Work out the finished part from the listing and answer in its coordinate system (mm). Face numbers are marked on the shaded views. A direction names the side the tool comes from. Coordinates: 2 decimals unless noted, no trailing zeros. Write each loop counter-clockwise with the first axis right and the second up, starting at its lowest first coordinate (ties: lowest second). Pieces come first, ordered by that corner, then holes. Notation, with made-up numbers: M -28.75,34.5 L 20.25,34.5 A24 ccw 20.25,61.5 Z; hole C 76.5,-4.75 d1. An arc over 180 degrees is marked long. Answer as CSV lines item,"result". Start each with the question number.
(1) The mould has two halves that part along X. Classify the marked faces 5, 6, 7 and 8: released by +X, released by -X, zero draft, split by the parting line, or undercut.
(2) Find the intervals of material crossed by L1, parallel to Y at x = -472, z = 61.5; L2, parallel to X at y = 260.5, z = 361; L3, parallel to Y at x = -29.5, z = 273, in increasing order. Write a range as [from, to].
(3) Flat-ended cylindrical pins translate along their axes: P1, Ø1.5, axis at x = -123.5, y = 183.5, coming from the -Z side; P2, Ø8, axis at x = -273.5, z = 408.5, coming from the +Y side; P3, Ø12, axis at y = 246.5, z = 200, coming from the +X side. Find the tip coordinate at first contact, or state that the pin passes through.
(4) For the marked faces 1, 2, 3 and 4, determine the directions among +Z, -Z, +X, -X, +Y, -Y from which every point of the face is accessible in a straight line to the end or side of a thin tool.
(5) A cutting plane is placed at D-D on x = -546. Give the vertices of the cut face in (y, z), then the cut area to 3 significant figures.
(6) A cutting plane is placed at A-A on z = 421. Give the vertices of the cut face in (x, y).
(7) A cutting plane is placed at B-B on y = 156.5. Give the vertices of the cut face in (x, z).
(8) A cutting plane is placed at C-C on x = -83. Give the vertices of the cut face in (y, z).
from build123d import *

# Parameters (mm, degrees)
F0_W      = 762
F0_H      = 457.2
F1_DEPTH  = 25.4
F2_W      = 50.8
F2_H      = 457.2
F3_DEPTH  = 25.4
F4_W      = 762
F4_H      = 457.2
F4_W_2    = 711.2
F4_H_2    = 406.4
F5_DEPTH  = 457.2
F6_W      = 50.8
F6_H      = 482.6
F7_DEPTH  = 25.4
F8_W      = 50.8
F8_H      = 482.6
F9_DEPTH  = 25.4
F10_W     = 76.2
F10_H     = 482.6
F11_DEPTH = 25.4
F12_W     = 76.2
F12_H     = 482.6
F13_DEPTH = 25.4
F15_DEPTH = 25.4


with BuildPart() as f1:
    # F0 (on Top) → F1 (new body)
    with BuildSketch(Plane.XY):
        with Locations((-381, 228.6)):
            Rectangle(F0_W, F0_H)
    extrude(amount=F1_DEPTH)

    # F2 (on face) → F3 (join)
    with BuildSketch(Plane(origin=(0, 0, 0), x_dir=(1, 0, 0), z_dir=(0, 0, -1))):
        with Locations((-584.2, -228.6)):
            Rectangle(F2_W, F2_H)
        with Locations((-177.8, -228.6)):
            Rectangle(F2_W, F2_H)
    extrude(amount=F3_DEPTH)

    # F4 (on face) → F5 (join)
    with BuildSketch(Plane.XY.offset(25.4)):
        with Locations((-381, 228.6)):
            Rectangle(F4_W, F4_H)
        with Locations((-381, 228.6)):
            Rectangle(F4_W_2, F4_H_2, mode=Mode.SUBTRACT)
    extrude(amount=F5_DEPTH)

    # F6 (on face) → F7 (join)
    with BuildSketch(Plane(origin=(0, 457.2, 0), x_dir=(-1, 0, 0), z_dir=(0, 1, 0))):
        with Locations((25.4, 241.3)):
            Rectangle(F6_W, F6_H)
        with Locations((736.6, 241.3)):
            Rectangle(F6_W, F6_H)
    extrude(amount=F7_DEPTH)

    # F8 (on face) → F9 (join)
    with BuildSketch(Plane.XZ):
        with Locations((-736.6, 241.3)):
            Rectangle(F8_W, F8_H)
        with Locations((-25.4, 241.3)):
            Rectangle(F8_W, F8_H)
    extrude(amount=F9_DEPTH)

    # F10 (on face) → F11 (join)
    with BuildSketch(Plane.YZ):
        with Locations((12.7, 241.3)):
            Rectangle(F10_W, F10_H)
        with Locations((444.5, 241.3)):
            Rectangle(F10_W, F10_H)
    extrude(amount=F11_DEPTH)

    # F12 (on face) → F13 (join)
    with BuildSketch(Plane(origin=(-762, 0, 0), x_dir=(0, -1, 0), z_dir=(-1, 0, 0))):
        with Locations((-444.5, 241.3)):
            Rectangle(F12_W, F12_H)
        with Locations((-12.7, 241.3)):
            Rectangle(F12_W, F12_H)
    extrude(amount=F13_DEPTH)

    # F14 (on face) → F15 (cut)
    with BuildSketch(Plane.XZ):
        with BuildLine():
            Line((-635, 482.6), (-635, 463.55))
            ThreePointArc((-635, 463.55), (-629.420384, 450.079616), (-615.95, 444.5))
            Line((-615.95, 444.5), (-146.05, 444.5))
            ThreePointArc((-146.05, 444.5), (-132.579616, 450.079616), (-127, 463.55))
            Line((-127, 463.55), (-127, 482.6))
            Line((-127, 482.6), (-635, 482.6))
        make_face()
    extrude(amount=-F15_DEPTH, mode=Mode.SUBTRACT)


solid = f1.part
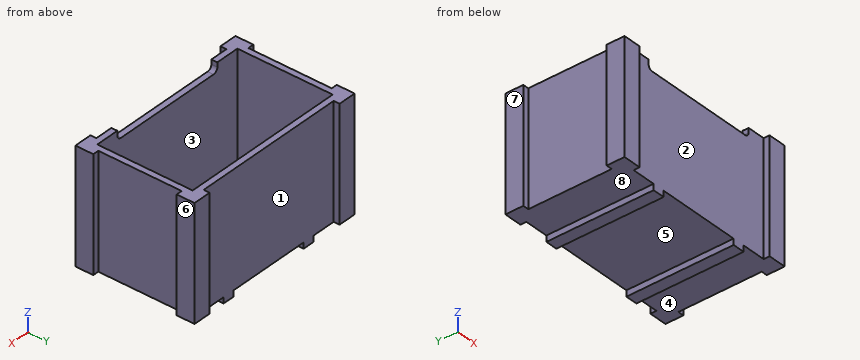
Here are the results:
1,face 5,"undercut"
1,face 6,"released by +X"
1,face 7,"released by -X"
1,face 8,"zero draft"
2,L1,"y = [0, 25.4], [431.8, 457.2]"
2,L2,"x = [-762, -736.6], [-25.4, 0]"
2,L3,"y = [-25.4, 25.4], [431.8, 482.6]"
3,P1,"stops at z = 0"
3,P2,"stops at y = 457.2"
3,P3,"stops at x = 0"
4,face 1,"+Z, -Z, +Y"
4,face 2,"+Z, -Z, -Y"
4,face 3,"+Z"
4,face 4,"-Z, +X, +Y, -Y"
5,outline,"M 0,0 L 457.2,0 L 457.2,482.6 L 431.8,482.6 L 431.8,25.4 L 25.4,25.4 L 25.4,444.5 L 0,444.5 Z"
5,area,"33,900 mm^2"
6,outline,"M -787.4,-25.4 L -711.2,-25.4 L -711.2,0 L -50.8,0 L -50.8,-25.4 L 25.4,-25.4 L 25.4,50.8 L 0,50.8 L 0,406.4 L 25.4,406.4 L 25.4,482.6 L -50.8,482.6 L -50.8,457.2 L -711.2,457.2 L -711.2,482.6 L -787.4,482.6 L -787.4,406.4 L -762,406.4 L -762,50.8 L -787.4,50.8 Z; hole M -736.6,25.4 L -25.4,25.4 L -25.4,431.8 L -736.6,431.8 Z"
7,outline,"M -762,0 L -609.6,0 L -609.6,-25.4 L -558.8,-25.4 L -558.8,0 L -203.2,0 L -203.2,-25.4 L -152.4,-25.4 L -152.4,0 L 0,0 L 0,482.6 L -25.4,482.6 L -25.4,25.4 L -736.6,25.4 L -736.6,482.6 L -762,482.6 Z"
8,outline,"M 0,0 L 457.2,0 L 457.2,482.6 L 431.8,482.6 L 431.8,25.4 L 25.4,25.4 L 25.4,482.6 L 0,482.6 Z"
